Autodesk Inventor part; units mm, degrees
ref_plane "YZ Plane" through (0, 0, 0) normal (1, 0, 0) x (0, 1, 0)
ref_plane "XZ Plane" through (0, 0, 0) normal (0, 1, 0) x (-1, 0, 0)
ref_plane "XY Plane" through (0, 0, 0) normal (0, 0, 1) x (1, 0, 0)
sketch "Sketch1" plane through (0, 0, 0) normal (0, 0, 1) x (1, 0, 0)
  line L0 (0, 0) -> (43, 0)
  line L1 (43, 0) -> (43, 20)
  line L2 (43, 20) -> (0, 20)
  line L3 (0, 20) -> (0, 0)
  dimension "d0" = 43
  dimension "d1" = 20
extrude "Extrusion1" add sketch "Sketch1" along normal blind 2
sketch "Sketch2" plane through (0, 0, 0) normal (0, -1, 0) x (1, 0, 0)
  line L0 (43, 0) -> (43, 2)
  line L1 (0, 0) -> (0, 2)
  line L2 (0, 0) -> (-2, 0)
  line L3 (-2, 0) -> (0, 2)
  line L4 (43, 0) -> (45, 0)
  line L5 (45, 0) -> (43, 2)
  dimension "d4" = 2
  dimension "d5" = 2
extrude "Extrusion2" add sketch "Sketch2" against normal blind 20
sketch "Sketch5" plane through (0, 0, 2) normal (0, 0, 1) x (1, 0, 0)
  line L0 (0, 0) -> (43, 0)
  line L1 (43, 20) -> (0, 20)
  line L2 (0, 20) -> (0, 0)
  line L3 (5, 5) -> (25, 5)
  line L4 (25, 5) -> (25, 15)
  line L5 (25, 15) -> (5, 15)
  line L6 (5, 15) -> (5, 5)
  dimension "d26" = 20
  dimension "d27" = 10
  dimension "d28" = 5
  dimension "d29" = 5
  dimension "d30" = 5
extrude "Extrusion5" cut sketch "Sketch5" against normal blind 1.5
sketch "Sketch6" plane through (5, 5, 2) normal (1, 0, 0) x (0, 0, -1)
  line L0 (0, 0) -> (0, 10)
  line L1 (0, 0) -> (1.5, 0)
  line L2 (1.5, 0) -> (1.5, 10)
  line L3 (0, 10) -> (1.5, 10)
  point P0 (2, -5)
extrude "Extrusion6" cut sketch "Sketch6" against normal up to next
sketch "Sketch7" plane through (0, 15, 2) normal (0, -1, 0) x (1, 0, 0)
  line L0 (0, 0) -> (25, 0)
  line L1 (-1.5, -1.5) -> (0, 0)
  line L2 (25, 0) -> (0, 0)
  line L3 (0, 0) -> (0, -0.5)
  line L4 (0, -0.5) -> (25, -0.5)
  line L5 (25, -0.5) -> (25, 0)
  line L6 (0, -0.5) -> (-0.5, -0.5)
  line L7 (0, 0) -> (-0.5, -0.5)
  point P0 (0, -2)
  dimension "d35" = 0.5
extrude "Extrusion7" add sketch "Sketch7" along normal blind 2
sketch "Sketch8" plane through (0, 5, 2) normal (0, 1, 0) x (1, 0, 0)
  line L0 (0, 0) -> (-1.5, 1.5)
  line L1 (25, 0) -> (0, 0)
  line L2 (0, 0) -> (0, 0.5)
  line L3 (0, 0.5) -> (25, 0.5)
  line L4 (25, 0.5) -> (25, 0)
  line L5 (0, 0.5) -> (-0.5, 0.5)
  line L6 (0, 0) -> (-0.5, 0.5)
  point P0 (0, 2)
  dimension "d38" = 25
  dimension "d39" = 0.5
extrude "Extrusion8" add sketch "Sketch8" along normal blind 2
chamfer "Chamfer1" distance 0.5 distance2 2 1 edges at (12.25, 7, 1.5) measured on face at (8.1667, 7, 1.6667)
chamfer "Chamfer2" distance 0.5 distance2 2 1 edges at (12.25, 13, 1.5) measured on face at (8.1667, 13, 1.6667)
properties part number "deksel token Edited"
Geometry check sheet. Reference: the model listing, model coordinates, mm. A direction names the side the tool comes from. Coordinates: 2 decimals unless noted, no trailing zeros. Write each loop counter-clockwise with the first axis right and the second up, starting at its lowest first coordinate (ties: lowest second). Pieces come first, ordered by that corner, then holes. Notation, with made-up numbers: M 35,67 L 69,67 A30 ccw 69,96 Z; hole C 62,26 d3. An arc over 180 degrees is marked long. Use one line per item in the form item = value. Start each with the question number.
1) Section check D-D on y = 2.5. Enter the section's corners in (x, z).
2) Section check B-B on y = 6. Enter the section's corners in (x, z), and give its area (3 significant figures).
3) Release check for a two-part mould opening along Y. For faces 3 (the flat face through (12.072, 5.986, 1.746)), 4 (the flat face through (22, 20, 1)), 5 (the flat face through (-1.7, 9.9, 0.3)) record: pulls with the +Y half, pulls with the -Y half, needs draft (parallel to the pull), parting line crosses it, or undercut.
4) Set-up check for faces 1 (the flat face through (21, 10, 0)), 2 (the flat face through (25, 10, 1)): record each of +Z, -Z, +X, -X, +Y, -Y from which the full face is reachable in a straight line by a thin tool's end or side.
5) Thickness scan on probe 1 along Y at (x, z) = (14, 1.3); probe 2 along Z at (x, y) = (3.5, 11.25); probe 3 along Z at (x, y) = (17.5, 5.75). Record the ranges inside material, lowest first. Write a range as from..to.
6) Go/stop test with flat-tipped pins: pin 1 Ø0.8 at (y, z) = (9, 1.5) entering from -X; pin 2 Ø1.5 at (x, y) = (15, 10.5) entering from +Z. Record where each tip stops, or that it passes through.
7) Section check C-C on y = 8.5. Enter the section's corners in (x, z).
Responses:
q1.outline = M -2,0 L 45,0 L 43,2 L 0,2 Z
q2.outline = M -2,0 L 45,0 L 43,2 L 0,2 L -0.25,1.75 L 25,1.75 L 25,0.5 L -1.5,0.5 Z
q2.area = 57.7 mm2
q3.face_3 = undercut
q3.face_4 = pulls with the +Y half
q3.face_5 = needs draft
q4.face_1 = -Z, +X, -X, +Y, -Y
q4.face_2 = -X
q5.probe_1 = 0..5, 15..20
q5.probe_2 = 0..0.5
q5.probe_3 = 0..0.5, 1.69..2
q6.pin_1 = 25
q6.pin_2 = 0.5
q7.outline = M -2,0 L 45,0 L 43,2 L 25,2 L 25,0.5 L -1.5,0.5 Z
